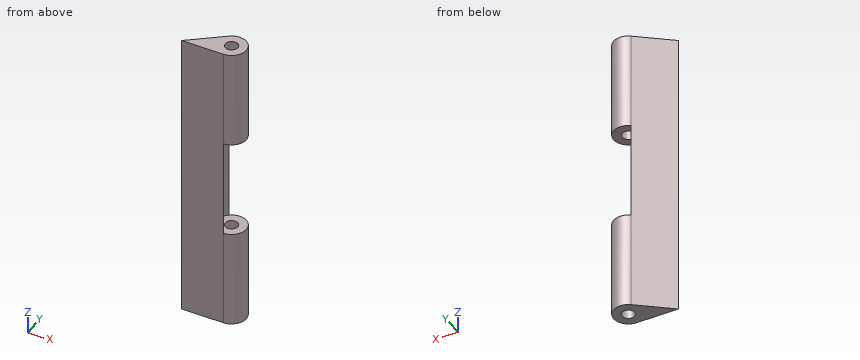
from build123d import *

# Parameters (mm, degrees)
SKETCH1_R           = 3.5
SKETCH1_R_2         = 1.5
BOSS_EXTRUDE1_DEPTH = 34.5
BOSS_EXTRUDE2_DEPTH = 34.5
SKETCH5_R           = 3.5
CUT_EXTRUDE1_DEPTH  = 11.5


with BuildPart() as part:
    # Sketch1 → Boss-Extrude1 (new, symmetric)
    with BuildSketch(Plane.XY):
        Circle(SKETCH1_R)
        Circle(SKETCH1_R_2, mode=Mode.SUBTRACT)
    extrude(amount=BOSS_EXTRUDE1_DEPTH, both=True)

    # Sketch2 → Boss-Extrude2 (add, symmetric)
    with BuildSketch(Plane.XY):
        with BuildLine():
            Line((0, -3.5), (-10, -3.5))
            Line((-10, -3.5), (-2.182628062, 2.736080178))
            ThreePointArc((-2.182628062, 2.736080178), (-3.303504247, -1.156226487), (0, -3.5))
        make_face()
    extrude(amount=BOSS_EXTRUDE2_DEPTH, both=True)

    # Sketch5 → Cut-Extrude1 (cut, symmetric)
    with BuildSketch(Plane.XY):
        Circle(SKETCH5_R)
    extrude(amount=CUT_EXTRUDE1_DEPTH, both=True, mode=Mode.SUBTRACT)


solid = part.part
The listing builds one solid part. Answer for the finished solid, in the listing's coordinates (mm). Give positions to 0.01 mm unless a question says otherwise; leave off trailing zeros. Loops run counter-clockwise (first coordinate to the right, second up) from the corner with the lowest first, then second, coordinate; pieces in that order, holes last. Notation, with made-up numbers: (50, 16.5) - (88, 16.5) arc R17 cw to (88, 41.5) - close; hole circle Ø6 at (50.25, -30.5). An arc over 180 degrees is marked (long way). Write each question's results on one line, items separated by ' | '.
1. Find section D-D, the plane x = -5. Write down the section's boundary in (y, z), then the cut area to 3 significant figures.
Resolved:
outline: (-3.5, -34.5) - (0.49, -34.5) - (0.49, 34.5) - (-3.5, 34.5) - close | area: 275 mm^2
2. Find section B-B, the plane y = 0. Write down the section's boundary in (x, z), then the cut area to 3 significant figures.
Resolved:
outline: (-5.61, -34.5) - (-1.5, -34.5) - (-1.5, -11.5) - (-3.5, -11.5) - (-3.5, 11.5) - (-1.5, 11.5) - (-1.5, 34.5) - (-5.61, 34.5) - close; (1.5, -34.5) - (3.5, -34.5) - (3.5, -11.5) - (1.5, -11.5) - close; (1.5, 11.5) - (3.5, 11.5) - (3.5, 34.5) - (1.5, 34.5) - close | area: 330 mm^2
3. Consider probe 1 along Z at (x, y) = (2, 2.75); probe 2 along Y at (x, z) = (0, -28.75); probe 3 along X at (y, z) = (0, 25.5). Determine where each line is inside the solid, lowest interval first. Write a range as from..to.
Resolved:
probe 1: z = -34.5..-11.5, 11.5..34.5 | probe 2: y = -3.5..-1.5, 1.5..3.5 | probe 3: x = -5.61..-1.5, 1.5..3.5
4. Find section A-A, the plane x = 2.5. Write down the section's boundary in (y, z), then the cut area to 3 significant figures.
Resolved:
outline: (-2.45, -34.5) - (2.45, -34.5) - (2.45, -11.5) - (-2.45, -11.5) - close; (-2.45, 11.5) - (2.45, 11.5) - (2.45, 34.5) - (-2.45, 34.5) - close | area: 225 mm^2
5. Find section C-C, the plane z = 14. Write down the section's boundary in (x, y), then the cut area to 3 significant figures.
Resolved:
outline: (-10, -3.5) - (0, -3.5) arc R3.5 ccw (long way) to (-2.18, 2.74) - close; hole circle Ø3 at (0, 0) | area: 51.3 mm^2
6. Flat-ended cylindrical pins translate along their axes: P1, Ø5, axis at x = -4.5, z = -13, coming from the +Y side; P2, Ø3, axis at x = -7.5, z = 25.5, coming from the +Y side; P3, Ø2.5, axis at x = 0, y = 0, coming from the +Z side; P4, Ø2, axis at x = -2, z = -23.5, coming from the +Y side. Find the tip coordinate at first contact, or state that the pin passes through.
Resolved:
P1: stops at y = 2.87 | P2: stops at y = -0.31 | P3: passes through | P4: stops at y = 3.35
